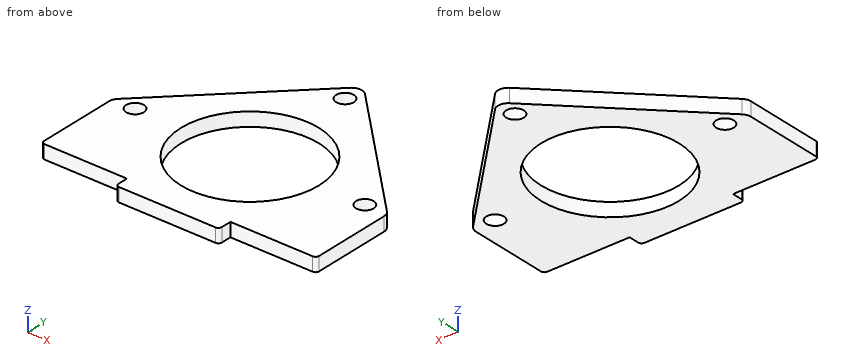
```python
from build123d import *

# Parameters (mm, degrees)
SKETCH_1_R      = 20
SKETCH_1_R_2    = 2.55
EXTRUDE_2_DEPTH = 4
FILLET_1_R      = 3
FILLET_2_R      = 1


with BuildPart() as part:
    # Эскиз1 → Бобышка-Вытянуть2 (new body)
    with BuildSketch(Plane.XY):
        Polygon((-39.880822459, 0), (0, 39.880822459), (39.880822459, 0), (39.880822459, -25), (15, -25), (15, -29), (-15, -29), (-15, -25), (-39.880822459, -25), align=None)
        Circle(SKETCH_1_R, mode=Mode.SUBTRACT)
        with Locations((-33.333013665, 0)):
            Circle(SKETCH_1_R_2, mode=Mode.SUBTRACT)
        with Locations((0, 33.333013665)):
            Circle(SKETCH_1_R_2, mode=Mode.SUBTRACT)
        with Locations((33.333013665, 0)):
            Circle(SKETCH_1_R_2, mode=Mode.SUBTRACT)
    extrude(amount=EXTRUDE_2_DEPTH)

    # Скругление1
    fillet_1_edges = [part.edges().sort_by_distance(p)[0] for p in [
        (-39.880822459, 0, 2),
        (0, 39.880822459, 2),
        (39.880822459, 0, 2),
    ]]
    fillet(fillet_1_edges, radius=FILLET_1_R)

    # Скругление2
    fillet_2_edges = [part.edges().sort_by_distance(p)[0] for p in [
        (39.880822459, -25, 2),
        (15, -29, 2),
        (-15, -29, 2),
        (-39.880822459, -25, 2),
    ]]
    fillet(fillet_2_edges, radius=FILLET_2_R)


solid = part.part
```
The listing builds one solid part. Answer for the finished solid, in the listing's coordinates (mm). Round coordinates to 2 decimals unless told otherwise and drop trailing zeros. Loops run counter-clockwise (first coordinate to the right, second up) from the corner with the lowest first, then second, coordinate; pieces in that order, holes last. Notation, with made-up numbers: (47.5, 36.5) - (72.5, 36.5) arc R6 cw to (72.5, 45.5) - close; hole circle Ø4 at (82, 39). An arc over 180 degrees is marked (long way). Use one line per item in the form item = value. Start each with the question number.
1. The part is cut by section A-A on x = 0. Determine the outline of the cut face in (y, z).
2. Given pin 1 Ø10 at (x, y) = (-23, 23.5) entering from -Z; pin 2 Ø2 at (x, z) = (21.5, 1.5) entering from -Y; pin 3 Ø3 at (x, y) = (-33.33, 0) entering from +Z; pin 4 Ø0.9 at (y, z) = (-26.5, 2) entering from -X, each flat-ended and moving along its own axis, determine where each tip first touches the part or whether it passes through.
3. Consider line 1 (Y direction, x = 0, z = 1.6); line 2 (Y direction, x = 0.5, z = 0.4); line 3 (X direction, y = -15.5, z = 0.6). Determine where each line is inside the solid, lowest interval first. Write a range as [from, to].
4. The part is cut by section B-B on x = 12. Determine the outline of the cut face in (y, z), then the cut area to 3 significant figures.
5. The part is cut by section C-C on y = 0. Determine the outline of the cut face in (x, z), then the cut area to 3 significant figures.
6. The part is cut by section D-D on z = 2.8. Determine the outline of the cut face in (x, y).
Geometry check:
q1.outline = (-29, 0) - (-20, 0) - (-20, 4) - (-29, 4) - close; (20, 0) - (30.78, 0) - (30.78, 4) - (20, 4) - close; (35.88, 0) - (38.64, 0) - (38.64, 4) - (35.88, 4) - close
q2.pin_1 = 0
q2.pin_2 = -25
q2.pin_3 = through
q2.pin_4 = -15
q3.line_1 = [-29, -20], [20, 30.78], [35.88, 38.64]
q3.line_2 = [-29, -19.99], [19.99, 30.83], [35.83, 38.6]
q3.line_3 = [-39.88, -12.64], [12.64, 39.88]
q4.outline = (-29, 0) - (-16, 0) - (-16, 4) - (-29, 4) - close; (16, 0) - (27.88, 0) - (27.88, 4) - (16, 4) - close
q4.area = 99.5 mm^2
q5.outline = (-39.61, 0) - (-35.88, 0) - (-35.88, 4) - (-39.61, 4) - close; (-30.78, 0) - (-20, 0) - (-20, 4) - (-30.78, 4) - close; (20, 0) - (30.78, 0) - (30.78, 4) - (20, 4) - close; (35.88, 0) - (39.61, 0) - (39.61, 4) - (35.88, 4) - close
q5.area = 116 mm^2
q6.outline = (-39.88, -24) arc R1 ccw to (-38.88, -25) - (-15, -25) - (-15, -28) arc R1 ccw to (-14, -29) - (14, -29) arc R1 ccw to (15, -28) - (15, -25) - (38.88, -25) arc R1 ccw to (39.88, -24) - (39.88, -1.24) arc R3 ccw to (39, 0.88) - (2.12, 37.76) arc R3 ccw to (-2.12, 37.76) - (-39, 0.88) arc R3 ccw to (-39.88, -1.24) - close; hole circle Ø5.1 at (-33.33, 0); hole circle Ø40 at (0, 0); hole circle Ø5.1 at (0, 33.33); hole circle Ø5.1 at (33.33, 0)
